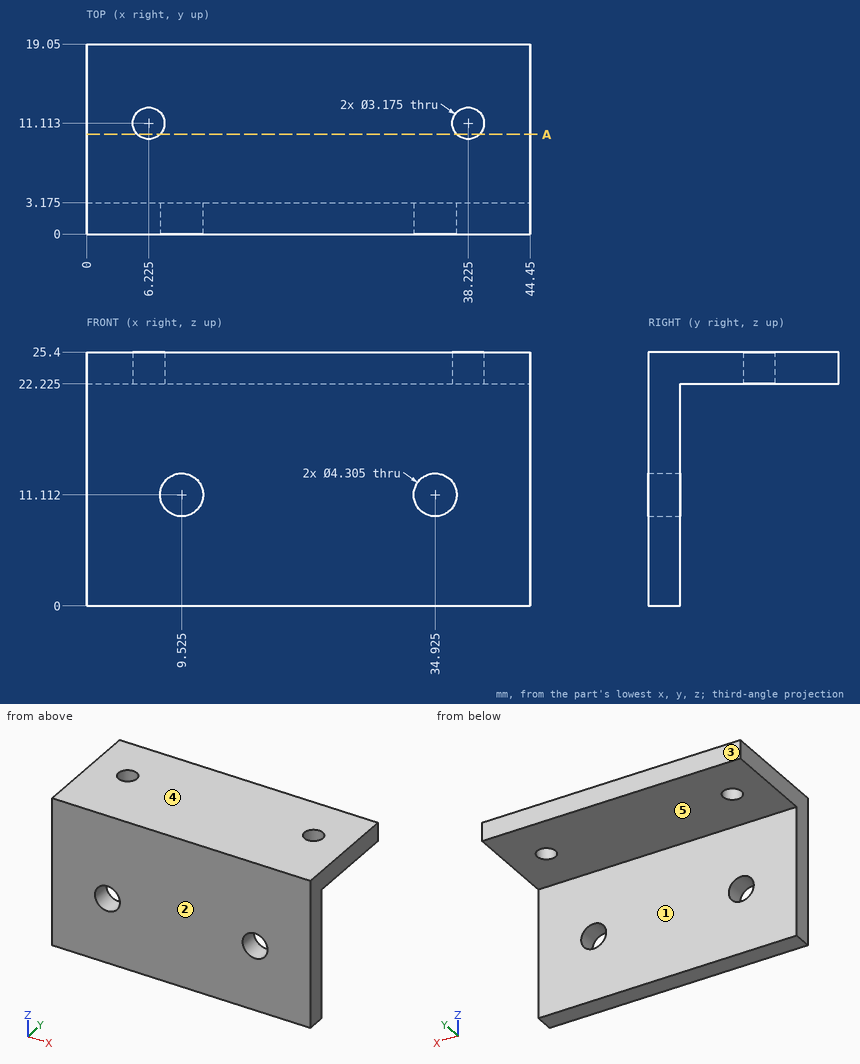
Design review of the part shown in the three views and the two pictorial views. Dimensions are in mm from the part's minimum x, y and z. A direction names the side the tool comes from. Round coordinates to 2 decimals unless told otherwise and drop trailing zeros. Use one line per item in the form item = value.
1) Clearance check with a flat-ended pin moving along its axis: pin 1 (11 mm diameter, centred on x = 23, z = 14, fed in from +Y) (1 decimal). State where the tip first meets the part, or that it passes through.
Found:
pin_1 = 3.2
2) Take a section at A-A, the plane y = 10. Count the separate pieces of the cut face and the enclosed holes in it, and give its area (3 significant figures).
Found:
separate_pieces = 3
enclosed_holes = 0
area = 127 mm2
3) Mouldability with a two-part tool opening along Z and no side actions: class the marked faces 3, 4 and 5 as +Z half, -Z half, draft (parallel to the pull), parting line (faces both ways), or undercut.
Found:
face_3 = draft
face_4 = +Z half
face_5 = -Z half
4) To check wall thickness, follow L1, parallel to Z at x = 22.5, y = 15.5 (1 decimal); L2, parallel to Y at x = 23, z = 9.5 (1 decimal); L3, parallel to X at y = 2, z = 10.75. State the ranges of each line that lie inside material, in increasing order. Write a range as from..to.
Found:
L1 = 22.2..25.4
L2 = 0..3.2
L3 = 0..7.4, 11.65..32.8, 37.05..44.45
5) Tool access review of the marked faces 1 and 2: name each direction out of +Z, -Z, +X, -X, +Y, -Y from which nothing blocks a thin tool from reaching the whole face with its end or side.
Found:
face_1 = -Z, +X, -X, +Y
face_2 = +Z, -Z, +X, -X, -Y
